Could you check a few things on this model? Use its own coordinates, in mm. Face numbers are marked on the shaded views. A direction names the side the tool comes from. Give positions to 0.01 mm unless a question says otherwise; leave off trailing zeros. Loops run counter-clockwise (first coordinate to the right, second up) from the corner with the lowest first, then second, coordinate; pieces in that order, holes last. Notation, with made-up numbers: (55, 47) -> (70, 47) arc R14 cw to (70, 70) -> close; hole circle Ø2 at (-17, -31.75). An arc over 180 degrees is marked (long way). Write item = value, one per line. Start each with the question number.
1) I need wall thicknesses on probe 1 along Y at (x, z) = (26.5, 8); probe 2 along X at (y, z) = (57.5, 6); probe 3 along Z at (x, y) = (38, 58). Which ranges of each line are inside material? Lowest first, please. Write a range as from..to.
2) On a 3-axis mill with a long thin cutter (end or side, diameter ignored), from which of +Z, -Z, +X, -X, +Y, -Y can I reach the whole of each face in a straight line? I mean the marked faces 1 and 2. Say none if no direction works.
3) I'm going to push flat-ended pins straight in: pin 1 Ø1 at (x, y) = (11, 55.5) entering from +Z; pin 2 Ø1.7 at (y, z) = (57.5, 5) entering from -X; pin 3 Ø1.7 at (x, z) = (17.5, 3) entering from -Y; pin 4 Ø1.7 at (y, z) = (60.5, 5) entering from +X. Where does each tip first touch, or does it pass through?
4) If we mould it in two halves opening along Y, with no side actions, what happens to the marked faces 3 and 4? For each: +Y half, -Y half, draft (parallel to the pull), parting line (faces both ways), or undercut.
5) I want a section at A-A (y = 56.5). List the corners of the cut face in (x, z) for me, and give its area (3 significant figures).
6) I want a section at D-D (x = 37). List the corners of the cut face in (y, z) for me.
7) I want a section at B-B (x = 32). List the corners of the cut face in (y, z) for me.
8) I want a section at C-C (z = 2.25). List the corners of the cut face in (x, y) for me.
Autodesk Fusion 360 part; units mm, degrees
sketch "Sketch1" plane through (0, 0, 0) normal (0, 0, 1) x (1, 0, 0)
  line L0 (0.4589, 72.3441) -> (40.8589, 72.3441)
  line L1 (40.8589, 72.3441) -> (40.8589, 42.9441)
  line L2 (40.8589, 42.9441) -> (0.4589, 42.9441)
  line L3 (0.4589, 42.9441) -> (0.4589, 72.3441)
  line L4 (7.7089, 61.5441) -> (33.6089, 61.5441)
  line L5 (33.6089, 61.5441) -> (33.6089, 53.7441)
  line L6 (33.6089, 53.7441) -> (7.7089, 53.7441)
  line L7 (7.7089, 53.7441) -> (7.7089, 61.5441)
  line L8 (20.6589, 72.3441) -> (20.6589, 42.9441) construction
  line L9 (7.7089, 57.6441) -> (33.6089, 57.6441) construction
  line L10 (35.6089, 51.7441) -> (5.7089, 51.7441)
  line L11 (5.7089, 51.7441) -> (5.7089, 63.5441)
  line L12 (5.7089, 63.5441) -> (35.6089, 63.5441)
  line L13 (35.6089, 63.5441) -> (35.6089, 51.7441)
  dimension "d7" = 10.8
  dimension "d8" = 10.8
  dimension "d9" = 7.8
  dimension "d10" = 25.9
  dimension "d11" = 40.4
  dimension "d12" = -2
extrude "Extrude1" add sketch "Sketch1" along normal blind 8.55 contours L10 L11 L12 L13
extrude "Extrude2" add sketch "Sketch1" along normal blind 1.5 contours L0 L1 L2 L3
sketch "Sketch2" plane through (0, 0, 8.55) normal (0, 0, 1) x (-1, 0, 0)
  line L0 (-33.6089, -53.7441) -> (-7.7089, -53.7441)
  line L1 (-7.7089, -53.7441) -> (-7.7089, -61.5441)
  line L2 (-7.7089, -61.5441) -> (-33.6089, -61.5441)
  line L3 (-33.6089, -61.5441) -> (-33.6089, -53.7441)
  line L4 (-35.6089, -63.5441) -> (-5.7089, -63.5441)
  line L5 (-5.7089, -63.5441) -> (-5.7089, -51.7441)
  line L6 (-5.7089, -51.7441) -> (-35.6089, -51.7441)
  line L7 (-35.6089, -51.7441) -> (-35.6089, -63.5441)
  line L8 (-40.8589, -72.3441) -> (-40.8589, -42.9441)
  line L9 (-0.4589, -72.3441) -> (-40.8589, -72.3441)
  line L10 (-40.8589, -42.9441) -> (-0.4589, -42.9441)
  line L11 (-0.4589, -42.9441) -> (-0.4589, -72.3441)
extrude "Extrude3" add sketch "Sketch2" against normal blind 1.5 contours L8 L9 L10 L11
equation "CenterLegWidth = 7.3 mm"
equation "CenterLegThickness = 25.4 mm"
equation "SideLegWidth = 3.65 mm"
equation "SideLegThickness = 25.4 mm"
equation "WindowWidth = 11.6 mm"
equation "WindowHeight = 9 mm"
equation "d7 = WindowWidth - 0.8 mm"
equation "d8 = WindowWidth - 0.8 mm"
equation "d9 = CenterLegWidth + 0.5 mm"
equation "d10 = CenterLegThickness + 0.5 mm"
equation "d11 = CenterLegThickness + 15 mm"
equation "d13 = WindowHeight - 0.45 mm"
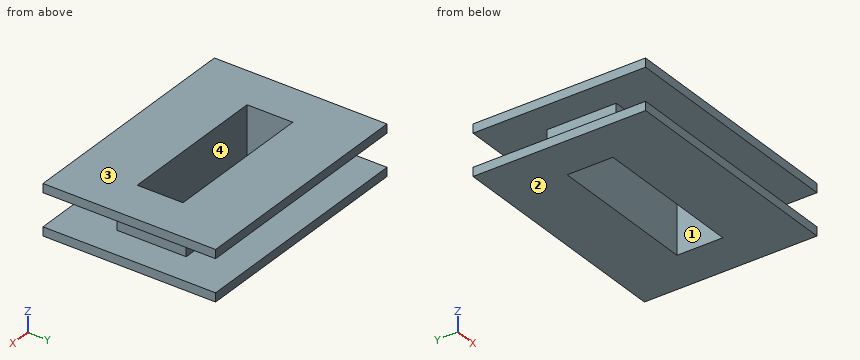
Answer list:
q1.probe_1 = 42.94..53.74, 61.54..72.34
q1.probe_2 = 5.71..7.71, 33.61..35.61
q1.probe_3 = 0..1.5, 7.05..8.55
q2.face_1 = +Z, -Z
q2.face_2 = -Z, +X, -X, +Y, -Y
q3.pin_1 = through
q3.pin_2 = 5.71
q3.pin_3 = 51.74
q3.pin_4 = 35.61
q4.face_3 = draft
q4.face_4 = undercut
q5.outline = (0.46, 0) -> (7.71, 0) -> (7.71, 8.55) -> (0.46, 8.55) -> (0.46, 7.05) -> (5.71, 7.05) -> (5.71, 1.5) -> (0.46, 1.5) -> close; (33.61, 0) -> (40.86, 0) -> (40.86, 1.5) -> (35.61, 1.5) -> (35.61, 7.05) -> (40.86, 7.05) -> (40.86, 8.55) -> (33.61, 8.55) -> close
q5.area = 65.7 mm^2
q6.outline = (42.94, 0) -> (72.34, 0) -> (72.34, 1.5) -> (42.94, 1.5) -> close; (42.94, 7.05) -> (72.34, 7.05) -> (72.34, 8.55) -> (42.94, 8.55) -> close
q7.outline = (42.94, 0) -> (53.74, 0) -> (53.74, 8.55) -> (42.94, 8.55) -> (42.94, 7.05) -> (51.74, 7.05) -> (51.74, 1.5) -> (42.94, 1.5) -> close; (61.54, 0) -> (72.34, 0) -> (72.34, 1.5) -> (63.54, 1.5) -> (63.54, 7.05) -> (72.34, 7.05) -> (72.34, 8.55) -> (61.54, 8.55) -> close
q8.outline = (5.71, 51.74) -> (35.61, 51.74) -> (35.61, 63.54) -> (5.71, 63.54) -> close; hole (7.71, 53.74) -> (33.61, 53.74) -> (33.61, 61.54) -> (7.71, 61.54) -> close
